```python
from build123d import *

# Parameters (mm, degrees)
ESBO_O1_W                = 50
ESBO_O1_H                = 50
RESSALTO_EXTRUS_O1_DEPTH = 130
ESBO_O2_W                = 25
ESBO_O2_H                = 3
RESSALTO_EXTRUS_O2_DEPTH = 70
ESBO_O4_W                = 17
ESBO_O4_H                = 17
RESSALTO_EXTRUS_O3_DEPTH = 17
ESBO_O5_R                = 4


with BuildPart() as part:
    # Esboço1 → Ressalto-extrusão1 (new body)
    with BuildSketch(Plane(origin=(0, 0, 0), x_dir=(1, 0, 0), z_dir=(0, 1, 0))):
        Rectangle(ESBO_O1_W, ESBO_O1_H)
    extrude(amount=RESSALTO_EXTRUS_O1_DEPTH)

    # Esboço2 → Ressalto-extrusão2 (add)
    with BuildSketch(Plane(origin=(25, 0, 0), x_dir=(0, 0, -1), z_dir=(1, 0, 0))):
        with Locations((0, 108.5)):
            Rectangle(ESBO_O2_W, ESBO_O2_H)
    extrude(amount=RESSALTO_EXTRUS_O2_DEPTH)

    # Esboço4 → Ressalto-extrusão3 (add)
    with BuildSketch(Plane(origin=(0, 110, 0), x_dir=(1, 0, 0), z_dir=(0, 1, 0))):
        with Locations((75, 0)):
            Rectangle(ESBO_O4_W, ESBO_O4_H)
    extrude(amount=RESSALTO_EXTRUS_O3_DEPTH)

    # Varredura1: sweep along a path in Esboço6
    with BuildLine(Plane(origin=(0, 0, 0), x_dir=(0, 0, -1), z_dir=(1, 0, 0))) as varredura1_path:
        Line((50, 170), (40, 170))
        ThreePointArc((40, 170), (11.715728753, 158.284271247), (0, 130))
    # Esboço5 → Varredura1 (sweep)
    with BuildSketch(Plane(origin=(0, 130, 0), x_dir=(1, 0, 0), z_dir=(0, 1, 0))):
        Circle(ESBO_O5_R)
    sweep(path=varredura1_path.line)


solid = part.part
```
Check sheet for the modelled part. Datum: model origin and axes. Units: mm. A direction names the side the tool comes from. Coordinates: 2 decimals unless noted, no trailing zeros. Loops run counter-clockwise (first coordinate to the right, second up) from the corner with the lowest first, then second, coordinate; pieces in that order, holes last. Notation, with made-up numbers: M 50,64.5 L 104,64.5 A23 ccw 104,88.5 Z; hole C -33.75,-6 d7. An arc over 180 degrees is marked long. Answer as a JSON object with one key per item and string values.
1. Scan lines: L1, parallel to Y at x = 62.5, z = 1; L2, parallel to X at y = 118, z = 14; L3, parallel to Y at x = -15, z = -9. Record each from-to range of solid material in increasing order. Write a range as from..to.
Outcome:
{"L1": "107..110", "L2": "-25..25", "L3": "0..130"}
2. Access from +Z, -Z, +X, -X, +Y, -Y to the whole of each face (thin tool, end or side, straight path). Record for faces 4 (the flat face through (75, 118, -8.5)), 5 (the flat face through (75, 127, 0)), 6 (the cylindrical face through (-0.521, 173.966, -44.93)), 7 (the flat face through (66.5, 118, 0)), 8 (the flat face through (60, 107, 0)).
Outcome:
{"face 4": "-Z, +X, +Y", "face 5": "+Z, -Z, +X, +Y", "face 6": "-Z", "face 7": "+Z, -Z, +Y", "face 8": "+Z, -Z, +X, -Y"}
3. Sectioned sample at C-C on x = 76. Record the cut outline in (y, z), and give its area (3 significant figures).
Outcome:
{"outline": "M 107,-12.5 L 110,-12.5 L 110,-8.5 L 127,-8.5 L 127,8.5 L 110,8.5 L 110,12.5 L 107,12.5 Z", "area": "364 mm²"}
4. Sectioned sample at D-D on x = 52. Record the cut outline in (y, z), and give its area (3 significant figures).
Outcome:
{"outline": "M 107,-12.5 L 110,-12.5 L 110,12.5 L 107,12.5 Z", "area": "75.0 mm²"}
5. Depth check by flat-ended pin: P1, Ø6, axis at x = 17, y = 131, coming from the -Z side; P2, Ø8, axis at x = 65, z = -15, coming from the +Y side; P3, Ø18.5, axis at y = 120, z = 1.5, coming from the +X side. Enter the tip coordinate at first touch or a pass-through.
Outcome:
{"P1": "z = -25", "P2": "y = 110", "P3": "x = 83.5"}
6. Release check for a two-part mould opening along X. For faces 1 (the flat face through (75, 118, 8.5)), 2 (the flat face through (52, 110, 0)), 3 (the flat face through (-25, 64, 0)) record: pulls with the +X half, pulls with the -X half, needs draft (parallel to the pull), parting line crosses it, or undercut.
Outcome:
{"face 1": "needs draft", "face 2": "undercut", "face 3": "pulls with the -X half"}
7. Sectioned sample at B-B on y = 47. Record the cut outline in (x, z).
Outcome:
{"outline": "M -25,-25 L 25,-25 L 25,25 L -25,25 Z"}
8. Sectioned sample at A-A on x = 0. Record the cut outline in (y, z), and give its area (3 significant figures).
Outcome:
{"outline": "M 0,-25 L 130,-25 L 130,-4 A36 cw 166,-40 L 166,-50 L 174,-50 L 174,-40 A44 ccw 130,4 L 130,25 L 0,25 Z", "area": "7,080 mm²"}
